Can you work these out from the drawing? Everything is in mm from the part's minimum corner. Round coordinates to 2 decimals unless told otherwise and drop trailing zeros. Write each loop counter-clockwise with the first axis right and the second up, starting at its lowest first coordinate (ties: lowest second). Pieces come first, ordered by that corner, then holes. Notation, with made-up numbers: (-32.5, 4.25) -> (-13.5, 4.25) arc R31 ccw to (-13.5, 42.25) -> close; hole circle Ø6 at (8.5, -38). An arc over 180 degrees is marked (long way). Write item = value, one per line. Start each with the question number.
1) Thinking about a two-plate mould opening in Y: for the marked faces 1, 2 and 3, which applies, +Y half, -Y half, draft (parallel to the pull), parting line (faces both ways), or undercut?
2) Imagine slicing it at A-A, the plane x = 25.5. Please give me the cut outline in (y, z).
3) If I drill on line 1 (X direction, y = 17.5, z = 10); line 2 (X direction, y = 20.5, z = 6.75) (1 decimal); line 3 (Y direction, x = 24.5, z = 8.25) (1 decimal), over which ranges is the centre line in solid material (lowest first)?
4) I'm going to push flat-ended pins straight in: pin 1 (1 mm diameter, centred on x = 18, z = 4, fed in from +Y); pin 2 (3 mm diameter, centred on y = 26.5, z = 9, fed in from +X); pin 3 (3 mm diameter, centred on x = 28, z = 4.5, fed in from -Y) (1 decimal). Where does each tip first touch, or does it pass through?
5) Imagine slicing it at D-D, the plane y = 29. Please give me the cut outline in (x, z), then the cut area to 3 significant figures.
6) Imagine slicing it at B-B, the plane y = 20. Please give me the cut outline in (x, z) (1 decimal).
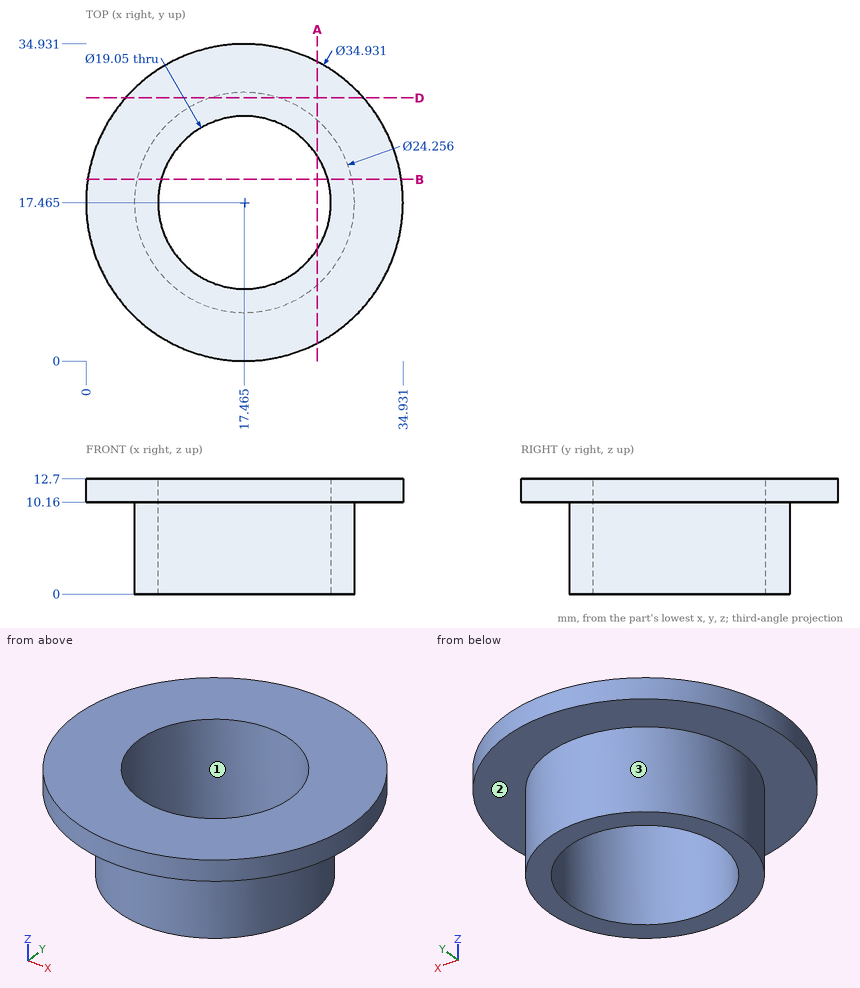
Reported:
q1.face_1 = undercut
q1.face_2 = draft
q1.face_3 = parting line
q2.outline = (1.96, 10.16) -> (8.38, 10.16) -> (8.38, 0) -> (12.35, 0) -> (12.35, 12.7) -> (1.96, 12.7) -> close; (22.58, 0) -> (26.55, 0) -> (26.55, 10.16) -> (32.97, 10.16) -> (32.97, 12.7) -> (22.58, 12.7) -> close
q3.line_1 = 5.34 to 7.94, 26.99 to 29.59
q3.line_2 = 5.7 to 8.4, 26.5 to 29.2
q3.line_3 = 7.6 to 11, 23.9 to 27.3
q4.pin_1 = 29.59
q4.pin_2 = 32.95
q4.pin_3 = 9.4
q5.outline = (4.35, 10.16) -> (13.72, 10.16) -> (13.72, 0) -> (21.21, 0) -> (21.21, 10.16) -> (30.58, 10.16) -> (30.58, 12.7) -> (4.35, 12.7) -> close
q5.area = 143 mm²
q6.outline = (0.2, 10.2) -> (5.6, 10.2) -> (5.6, 0) -> (8.3, 0) -> (8.3, 12.7) -> (0.2, 12.7) -> close; (26.6, 0) -> (29.3, 0) -> (29.3, 10.2) -> (34.7, 10.2) -> (34.7, 12.7) -> (26.6, 12.7) -> close
